```python
from build123d import *

# Parameters (mm, degrees)
BOSS_EXTRUDE1_DEPTH = 8.937498
SKETCH2_W           = 4
SKETCH2_H           = 4
BOSS_EXTRUDE4_DEPTH = 8.937498
SKETCH3_W           = 4
SKETCH3_H           = 4
BOSS_EXTRUDE5_DEPTH = 11.9375
FILLET1_R           = 4
SKETCH4_R           = 0.9
CUT_EXTRUDE1_DEPTH  = 6


with BuildPart() as part:
    # Sketch1 → Boss-Extrude1 (new body)
    with BuildSketch(Plane(origin=(0, 0, 0), x_dir=(1, 0, 0), z_dir=(0, 1, 0))):
        Polygon((8.937498, 8.937498), (0, 8.937498), (0, 1), (-3, 1), (-3, -3), (1, -3), (1, 0), (8.937498, 0), align=None)
    extrude(amount=BOSS_EXTRUDE1_DEPTH)

    # Sketch2 → Boss-Extrude4 (add)
    with BuildSketch(Plane.XY):
        with Locations((-1, -1)):
            Rectangle(SKETCH2_W, SKETCH2_H)
    extrude(amount=-BOSS_EXTRUDE4_DEPTH)

    # Sketch3 → Boss-Extrude5 (add)
    with BuildSketch(Plane.ZY.offset(3)):
        with Locations((1, -1)):
            Rectangle(SKETCH3_W, SKETCH3_H)
    extrude(amount=-BOSS_EXTRUDE5_DEPTH)

    # Fillet1
    fillet1_edges = [part.edges().sort_by_distance(p)[0] for p in [
        (-3, -3, -2.968749),
        (2.96875, -3, 3),
        (-3, 2.968749, 3),
    ]]
    fillet(fillet1_edges, radius=FILLET1_R - 0.0001)  # a hair under: the kernel refuses the full size

    # Sketch4 → Cut-Extrude1 (cut)
    with BuildSketch(Plane.XZ):
        with Locations(Location((4.968749, -4.968749, 0), (0, 0, 270))):
            Circle(SKETCH4_R)
    extrude(amount=-CUT_EXTRUDE1_DEPTH, mode=Mode.SUBTRACT)


solid = part.part
```
Build history of the part. All positions in model axes, mm. A direction names the side the tool comes from. Round coordinates to 2 decimals unless told otherwise and drop trailing zeros. Write each loop counter-clockwise with the first axis right and the second up, starting at its lowest first coordinate (ties: lowest second). Pieces come first, ordered by that corner, then holes. Notation, with made-up numbers: (-16.75, -39.5) -> (41.25, -39.5) arc R32 ccw to (41.25, -6.5) -> close; hole circle Ø5 at (-23, 52). An arc over 180 degrees is marked (long way). Put each result on its own line as item: value.
Item 1: Two-plate mould, pull along Z, no slides. Class faces 1 (the face through (-2, 1, -5)), 2 (the face through (5, 5, 0)), 3 (the face through (4.421, 2.958, -4.255)): pulls with the +Z half, pulls with the -Z half, needs draft (parallel to the pull), parting line crosses it, or undercut.
Here are the results:
face 1: needs draft
face 2: pulls with the +Z half
face 3: undercut
Item 2: Slice it at D-D, the plane y = -0.75. Give the cut face in (x, z), plus the area to 3 significant figures.
Here are the results:
outline: (-2.6, -8.94) -> (1, -8.94) -> (1, -1) -> (8.94, -1) -> (8.94, 2.6) -> (1, 2.6) arc R3.6 ccw to (-2.6, -1) -> close
area: 67.3 mm^2
Item 3: Wall check: probe 1 along Y at (x, z) = (1.25, -6); probe 2 along Z at (x, y) = (4.75, 4.75). Give the ranges that are in metal, low to high. Write a range as from..to.
Here are the results:
probe 1: y = 0..8.94
probe 2: z = -8.94..-5.84, -4.1..0
Item 4: Tool access for faces 4 (the face through (-1, 5, -1)), 5 (the face through (1, 5, 2)), 6 (the face through (4, 0, -6)), 7 (the face through (5.024, -1.859, 1.797)): list every direction of +Z, -Z, +X, -X, +Y, -Y with a clear straight run to the whole face (end or side of a thin tool).
Here are the results:
face 4: -Z, -X, +Y
face 5: +Z, +X, +Y
face 6: -Z, +X, -Y
face 7: +Z, +X, -X, -Y
Item 5: Flat gauge pins, fed straight in: P1, Ø2.5, axis at y = 5.5, z = -4.5, coming from the -X side; P2, Ø1.2, axis at x = 6.5, y = -1, coming from the -Z side; P3, Ø0.5, axis at x = 5, z = -5, coming from the -Y side. Where does each tip first touch, or does it go through?
Here are the results:
P1: stops at x = 0
P2: stops at z = -1
P3: stops at y = 6
